Can you work these out from the model? Positions are in its coordinate system, mm. A direction names the side the tool comes from. Coordinates: 2 decimals unless noted, no trailing zeros. Loops run counter-clockwise (first coordinate to the right, second up) from the corner with the lowest first, then second, coordinate; pieces in that order, holes last. Notation, with made-up numbers: (63.25, 27) -> (100.25, 27) arc R5 ccw to (100.25, 36) -> close; hole circle Ø11 at (-9.75, 78). An arc over 180 degrees is marked (long way). Use one line per item in the form item = value. Start each with the question number.
(1) Thinking about a two-plate mould opening in X: for faces 1 (the cylindrical face through (9.09, -22.66, 2.54)), 2 (the cylindrical face through (-1.08, -4.88, 2.53)), 3 (the cylindrical face through (3.461, -126.654, 6.041)), which applies, released by +X, released by -X, zero draft, split by the parting line, or undercut?
(2) On a 3-axis mill with a long thin cutter (end or side, diameter ignored), from which of +Z, -Z, +X, -X, +Y, -Y can I reach the whole of each face in a straight line? I mean faces 4 (the flat face through (0, -55, 0)), 5 (the flat face through (7.5, -79, 2)), 6 (the flat face through (-7.5, -81, 2)), 7 (the flat face through (0, -120, 30)), 8 (the flat face through (2, -125, 10)). Say none if no direction works.
(3) I need wall thicknesses on line 1 (Z direction, x = 1, y = -52); line 2 (Y direction, x = -0.5, z = 17.75); line 3 (Y direction, x = 3.5, z = 11.75). Which ranges of each line are inside material? Lowest first, please. Write a range as [from, to].
(4) Imagine slicing it at D-D (z = 23.75). List the corners of the cut face in (x, y) for me.
(5) Imagine slicing it at B-B (x = 1.5). List the corners of the cut face in (y, z) for me, plus the area to 3 significant figures.
(6) I'm going to push flat-ended pins straight in: pin 1 (6 mm diameter, centred on x = -1.5, z = 21, fed in from +Y); pin 2 (1.5 mm diameter, centred on x = -8.5, z = 3, fed in from +Y); pin 3 (9 mm diameter, centred on x = -4.5, y = -64, fed in from +Z). Where does each tip first touch, or does it pass through?
(7) Imagine slicing it at C-C (y = -45). List the corners of the cut face in (x, z) for me.
(8) Imagine slicing it at A-A (y = 0). List the corners of the cut face in (x, z) for me, plus the area to 3 significant figures.
```python
from build123d import *

# Parameters (mm, degrees)
BOSS_EXTRUDE1_DEPTH            = 5
SKETCH2_R                      = 7.5
BOSS_EXTRUDE2_DEPTH            = 5
SKETCH3_R                      = 5
BOSS_EXTRUDE3_DEPTH            = 20
F_10_0_10_DIAMETER_HOLE1_D     = 10
F_10_0_10_DIAMETER_HOLE1_DEPTH = 30
FILLET1_R                      = 95.416666667


with BuildPart() as part:
    # Sketch1 → Boss-Extrude1 (new body)
    with BuildSketch(Plane(origin=(0, 0, 0), x_dir=(-1, 0, 0), z_dir=(0, 0, -1))):
        with BuildLine():
            Line((7.499999998, -120), (7.499999998, -12.990381057))
            ThreePointArc((7.499999998, -12.990381057), (-1e-09, 15.000000001), (-7.5, -12.990381057))
            Line((-7.5, -12.990381057), (-7.5, -120))
            ThreePointArc((-7.5, -120), (-1e-09, -127.499999999), (7.499999998, -120))
        make_face()
    extrude(amount=-BOSS_EXTRUDE1_DEPTH)

    # Sketch2 → Boss-Extrude2 (add)
    with BuildSketch(Plane.XY.offset(5)):
        with Locations((0, -120)):
            Circle(SKETCH2_R)
    extrude(amount=BOSS_EXTRUDE2_DEPTH)

    # Sketch3 → Boss-Extrude3 (add)
    with BuildSketch(Plane.XY.offset(10)):
        with Locations((0, -120)):
            Circle(SKETCH3_R)
    extrude(amount=BOSS_EXTRUDE3_DEPTH)

    # Ø10.0 (10) Diameter Hole1
    with Locations(Plane(origin=(0, 0, 0), x_dir=(-1, 0, 0), z_dir=(0, 0, -1))):
        with Locations((0, 0)):
            Hole(F_10_0_10_DIAMETER_HOLE1_D / 2, depth=F_10_0_10_DIAMETER_HOLE1_DEPTH)

    # Fillet1
    fillet1_edges = [part.edges().sort_by_distance(p)[0] for p in [
        (7.5, -12.990381057, 2.5),
        (-7.499999998, -12.990381057, 2.5),
    ]]
    fillet(fillet1_edges, radius=FILLET1_R)


solid = part.part
```
Worked out:
q1.face_1 = released by +X
q1.face_2 = undercut
q1.face_3 = split by the parting line
q2.face_4 = -Z, +X, -X, +Y, -Y
q2.face_5 = +Z, -Z, +X, -Y
q2.face_6 = +Z, -Z, -X, -Y
q2.face_7 = +Z, +X, -X, +Y, -Y
q2.face_8 = +Z
q3.line_1 = [0, 5]
q3.line_2 = [-124.97, -115.03]
q3.line_3 = [-123.57, -116.43]
q4.outline = circle Ø10 at (0, -120)
q5.outline = (-127.35, 0) -> (-4.77, 0) -> (-4.77, 5) -> (-112.65, 5) -> (-112.65, 10) -> (-115.23, 10) -> (-115.23, 30) -> (-124.77, 30) -> (-124.77, 10) -> (-127.35, 10) -> close; (4.77, 0) -> (14.92, 0) -> (14.92, 5) -> (4.77, 5) -> close
q5.area = 928 mm2
q6.pin_1 = -115
q6.pin_2 = 12.84
q6.pin_3 = 5
q7.outline = (-7.5, 0) -> (7.5, 0) -> (7.5, 5) -> (-7.5, 5) -> close
q8.outline = (-15, 0) -> (-5, 0) -> (-5, 5) -> (-15, 5) -> close; (5, 0) -> (15, 0) -> (15, 5) -> (5, 5) -> close
q8.area = 100 mm2
